Geometry: final body of the model. Coordinates: model frame, mm. A direction names the side the tool comes from. Coordinates: 2 decimals unless noted, no trailing zeros. Loops run counter-clockwise (first coordinate to the right, second up) from the corner with the lowest first, then second, coordinate; pieces in that order, holes last. Notation, with made-up numbers: (-14, 35) - (0, 35) arc R22 ccw to (0, 68) - close; hole circle Ø4 at (64.25, 49). An arc over 180 degrees is marked (long way). Answer in a Markdown table with one row per item.
from build123d import *

# Parameters (mm, degrees)
ESQUISSE1_W                      = 32
ESQUISSE1_H                      = 7.5
ESQUISSE2_R                      = 2.5
ENL_V_MAT_EXTRU_1_DEPTH          = 22
ESQUISSE4_R                      = 4
ENL_V_MAT_EXTRU_2_DEPTH          = 6
D_GAGEMENT_M1_41_D               = 1.6
D_GAGEMENT_M1_41_DEPTH           = 6
D_GAGEMENT_M1_41_TIP             = 0.480688495
D_GAGEMENT_M1_41_ON_FACE_2_D     = 1.6
D_GAGEMENT_M1_41_ON_FACE_2_DEPTH = 6
D_GAGEMENT_M1_41_ON_FACE_2_TIP   = 0.480688495


with BuildPart() as part:
    # Esquisse1 → Révolution2 (revolve)
    with BuildSketch(Plane.XY, mode=Mode.PRIVATE) as r_volution2_sk:
        with Locations((16, 3.75)):
            Rectangle(ESQUISSE1_W, ESQUISSE1_H)
    revolve(r_volution2_sk.sketch.rotate(Axis((0, 7.5, 0), (1, 0, 0)), 270), axis=Axis((0, 7.5, 0), (1, 0, 0)))

    # Esquisse2 → Enlèv. mat.-Extru.1 (cut)
    with BuildSketch(Plane(origin=(32, 0, 0), x_dir=(0, 0, -1), z_dir=(1, 0, 0))):
        with Locations((0, 7.5)):
            Circle(ESQUISSE2_R)
    extrude(amount=-ENL_V_MAT_EXTRU_1_DEPTH, mode=Mode.SUBTRACT)

    # Esquisse4 → Enlèv. mat.-Extru.2 (cut)
    with BuildSketch(Plane.ZY):
        with Locations((0, 7.5)):
            Circle(ESQUISSE4_R)
    extrude(amount=-ENL_V_MAT_EXTRU_2_DEPTH, mode=Mode.SUBTRACT)

    # Dégagement M1.41
    with Locations(Plane(origin=(21.894837685, 0.022480062, -0.580254755), x_dir=(0, 0.077367300627, -0.997002658368), z_dir=(0, -0.997002658368, -0.077367300627))):
        with Locations((0, 0)):
            Hole(D_GAGEMENT_M1_41_D / 2, depth=D_GAGEMENT_M1_41_DEPTH)
            with Locations((0, 0, -(D_GAGEMENT_M1_41_DEPTH + D_GAGEMENT_M1_41_TIP / 2))):  # 118° drill point
                Cone(0, D_GAGEMENT_M1_41_D / 2, D_GAGEMENT_M1_41_TIP, mode=Mode.SUBTRACT)

    # Dégagement M1.41 on face 2
    with Locations(Plane(origin=(12.788839851, 0.005106148, -0.276705898), x_dir=(0, 0.036894006807, -0.999319184376), z_dir=(0, -0.999319184376, -0.036894006807))):
        with Locations((0, 0)):
            Hole(D_GAGEMENT_M1_41_ON_FACE_2_D / 2, depth=D_GAGEMENT_M1_41_ON_FACE_2_DEPTH)
            with Locations((0, 0, -(D_GAGEMENT_M1_41_ON_FACE_2_DEPTH + D_GAGEMENT_M1_41_ON_FACE_2_TIP / 2))):  # 118° drill point
                Cone(0, D_GAGEMENT_M1_41_ON_FACE_2_D / 2, D_GAGEMENT_M1_41_ON_FACE_2_TIP, mode=Mode.SUBTRACT)


solid = part.part
(1) Cut plane C-C on z = -4.5. Output: boundary loops of the cut face in (x, y), then the cut area to 3 significant figures.
Verdict:
| item | result |
|---|---|
| outline | (0, 1.5) - (32, 1.5) - (32, 13.5) - (0, 13.5) - close |
| area | 384 mm² |
(2) Ray query, probe 1 along Y at (x, z) = (15, 0); probe 2 along Y at (x, z) = (3, 0); probe 3 along X at (y, z) = (9.75, -1.5). Return the intervals inside material, ascending.
Verdict:
| item | result |
|---|---|
| probe 1 | y = 0 to 5, 10 to 15 |
| probe 2 | y = 0 to 3.5, 11.5 to 15 |
| probe 3 | x = 6 to 32 |
(3) Cut plane A-A on y = 7.5. Output: boundary loops of the cut face in (x, z), then the cut area to 3 significant figures.
Verdict:
| item | result |
|---|---|
| outline | (0, -7.5) - (32, -7.5) - (32, -2.5) - (10, -2.5) - (10, 2.5) - (32, 2.5) - (32, 7.5) - (0, 7.5) - (0, 4) - (6, 4) - (6, -4) - (0, -4) - close |
| area | 322 mm² |
(4) Pull-direction query (Z, two-part tool) for faces 1 (the face through (22.57, 2.59, 0.05)), 2 (the face through (16.22, 14.82, -1.63)), 3 (the face through (0, 11, 3)); classes: pulls with the +Z half, pulls with the -Z half, needs draft (parallel to the pull), parting line crosses it, or undercut.
Verdict:
| item | result |
|---|---|
| face 1 | undercut |
| face 2 | parting line crosses it |
| face 3 | needs draft |
(5) First-contact query: pin 1 Ø1.5 at (x, z) = (19, -1) entering from +Y; pin 2 Ø3 at (x, y) = (21.5, 5) entering from +Z; pin 3 Ø1 at (y, z) = (9, 2.5) entering from -X; pin 4 Ø4 at (y, z) = (7.5, -1) entering from +X. Flat tips, straight axial feed; report the tip coordinate or a pass-through.
Verdict:
| item | result |
|---|---|
| pin 1 | stops at y = 15 |
| pin 2 | stops at z = 7.43 |
| pin 3 | stops at x = 6 |
| pin 4 | stops at x = 32 |
(6) Access query for faces 4 (the face through (10, 8, 0)), 5 (the face through (2.958, 3.595, -0.867)), 6 (the face through (12.302, 2.631, -0.815)). Directions: +Z, -Z, +X, -X, +Y, -Y. A direction counts if a zero-diameter tool reaches every point of the face in a straight line with its end or side. Return the directions, or none.
Verdict:
| item | result |
|---|---|
| face 4 | +X |
| face 5 | -X |
| face 6 | none |
(7) Cut plane B-B on x = 15. Output: boundary loops of the cut face in (y, z).
Verdict:
| item | result |
|---|---|
| outline | circle Ø15 at (7.5, 0); hole circle Ø5 at (7.5, 0) |
(8) Cut plane D-D on x = 9. Output: boundary loops of the cut face in (y, z), then the cut area to 3 significant figures.
Verdict:
| item | result |
|---|---|
| outline | circle Ø15 at (7.5, 0) |
| area | 177 mm² |
